The listing builds one solid part. Answer for the finished solid, in the listing's coordinates (mm). A direction names the side the tool comes from. Round coordinates to 2 decimals unless told otherwise and drop trailing zeros. Write each loop counter-clockwise with the first axis right and the second up, starting at its lowest first coordinate (ties: lowest second). Pieces come first, ordered by that corner, then holes. Notation, with made-up numbers: (68, 8) -> (81, 8) arc R16 ccw to (81, 33) -> close; hole circle Ø4 at (84, 67). An arc over 180 degrees is marked (long way). Write each question's results on one line, items separated by ' | '. Start each with the question number.
```python
from build123d import *

# Parameters (mm, degrees)
F1_DEPTH = 63.5
F0_W     = 25.4
F0_H     = 19.05
F2_DEPTH = 25.4
F3_DEPTH = 7.9375


# Not quite as in the source:
# - the program builds the solid bodies; features that only make, move or delete a surface that nothing else refers to are left out


with BuildPart() as f1:
    # F0 (on Front) → F1 (new body, symmetric)
    with BuildSketch(Plane.XZ):
        Polygon((38.861105454, 9.525), (-57.911105454, 9.525), (-57.911105454, -9.525), (57.911105454, -9.525), (57.911105454, 9.525), align=None)
    extrude(amount=F1_DEPTH, both=True)

    # F0 (on Front) → F2 (join, symmetric)
    with BuildSketch(Plane.XZ):
        with BuildLine():
            Line((38.861105454, 27.0002), (38.861105454, 9.525))
            Line((38.861105454, 9.525), (57.911105454, 9.525))
            Line((57.911105454, 9.525), (57.911105454, 27.0002))
            ThreePointArc((57.911105454, 27.0002), (62.5607853026, 38.2255201513), (73.786105454, 42.8752))
            Line((73.786105454, 42.8752), (76.961105454, 42.8752))
            Line((76.961105454, 42.8752), (76.961105454, 61.9252))
            Line((76.961105454, 61.9252), (73.786105454, 61.9252))
            add(Edge.make_bspline(
                [(71.3194409243, 61.8379839579), (72.1527081081, 61.872613516), (72.9751435191, 61.9016976168), (73.786105454, 61.9252)],
                knots=[139.2706883943, 139.2706883943, 139.2706883943, 139.2706883943, 141.7389724845, 141.7389724845, 141.7389724845, 141.7389724845], degree=3))
            ThreePointArc((71.3194409243, 61.8379839579), (48.2331811233, 50.8078391763), (38.861105454, 27.0002))
        make_face()
        with Locations((89.661105454, 52.4002)):
            Rectangle(F0_W, F0_H)
    extrude(amount=F2_DEPTH, both=True)

    # F0 (on Front) → F3 (join, symmetric)
    with BuildSketch(Plane.XZ):
        with BuildLine():
            add(Edge.make_bspline(
                [(-57.911105454, 9.525), (-57.1981257704, 40.2751503058), (24.3030967511, 59.8840425909), (71.3194409243, 61.8379839579)],
                knots=[0, 0, 0, 0, 139.2706883943, 139.2706883943, 139.2706883943, 139.2706883943], degree=3))
            Line((-57.911105454, 9.525), (38.861105454, 9.525))
            Line((38.861105454, 9.525), (38.861105454, 27.0002))
            ThreePointArc((38.861105454, 27.0002), (48.2331811233, 50.8078391763), (71.3194409243, 61.8379839579))
        make_face()
    extrude(amount=F3_DEPTH, both=True)


solid = f1.part
```
Q1. For faces 1 (the flat face through (63, -25.4, 42)), 2 (the flat face through (63, 25.4, 42)), 3 (the flat face through (8, 7.938, 30)), 4 (the flat face through (57.911, -1, 4)), 5 (the flat face through (8, -7.938, 30)), determine the directions among +Z, -Z, +X, -X, +Y, -Y from which every point of the face is accessible in a straight line to the end or side of a thin tool.
Q2. The part is cut by section A-A, the plane y = 27.5. Write down the section's boundary in (x, z) (3 decimals).
Q3. Each of these flat-tipped pins is pushed along its axis until it touches: pin 1 (15.5 mm diameter, centred on x = 13, z = 28, fed in from +Y); pin 2 (8.5 mm diameter, centred on y = 15.5, z = 15, fed in from -X); pin 3 (11 mm diameter, centred on y = 28.5, z = 5, fed in from +X). Where does it stop, or does it pass through?
Q4. Find the intervals of material crossed by line 1 (Z direction, x = 23.5, y = -38) (3 decimals); line 2 (X direction, y = -53, z = 0); line 3 (Y direction, x = 94.5, z = 57), in increasing order.
Answers follow:
1) face 1: +Z, +X, -X, -Y | face 2: +Z, +X, -X, +Y | face 3: +Z, -X, +Y | face 4: -Z, +X, +Y, -Y | face 5: +Z, -X, -Y
2) outline: (-57.911, -9.525) -> (57.911, -9.525) -> (57.911, 9.525) -> (-57.911, 9.525) -> close
3) pin 1: y = 7.94 | pin 2: x = 38.86 | pin 3: x = 57.91
4) line 1: -9.525 to 9.525 | line 2: -57.91 to 57.91 | line 3: -25.4 to 25.4
